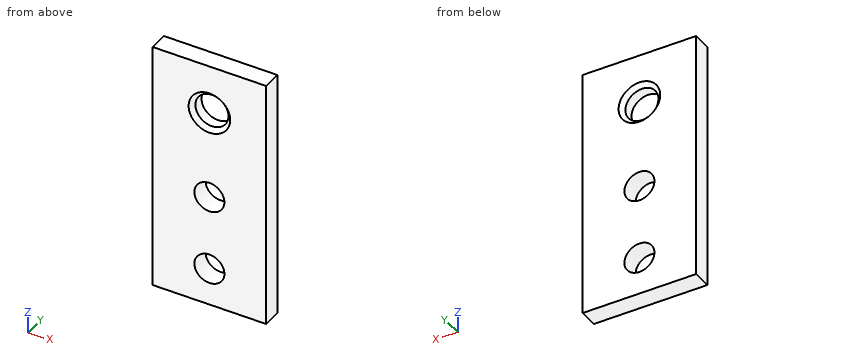
```python
from build123d import *

# Parameters (mm, degrees)
SKETCH1_W                   = 38.1
SKETCH1_H                   = 6.35
EXTRUDE1_DEPTH              = 84.455
F_3_8_CLEARANCE_HOLE1_D     = 10.0838
F_3_8_CLEARANCE_HOLE1_DEPTH = 16.002
F_3_8_CLEARANCE_HOLE1_TIP   = 3.029479155


with BuildPart() as part:
    # Sketch1 → Extrude1 (new body)
    with BuildSketch(Plane.XY):
        Rectangle(SKETCH1_W, SKETCH1_H)
    extrude(amount=EXTRUDE1_DEPTH)

    # 3/8 Clearance Hole1
    with Locations(Plane(origin=(0, 3.175, 12.7), x_dir=(0, 0, 1), z_dir=(0, 1, 0))):
        with Locations((0, 0), (25.4, 0)):
            Hole(F_3_8_CLEARANCE_HOLE1_D / 2, depth=F_3_8_CLEARANCE_HOLE1_DEPTH)
            with Locations((0, 0, -(F_3_8_CLEARANCE_HOLE1_DEPTH + F_3_8_CLEARANCE_HOLE1_TIP / 2))):  # 118° drill point
                Cone(0, F_3_8_CLEARANCE_HOLE1_D / 2, F_3_8_CLEARANCE_HOLE1_TIP, mode=Mode.SUBTRACT)

    # Sketch4 → 7/16 (0.4375) Diameter Hole2 (revolve, cut)
    with BuildSketch(Plane(origin=(0, 3.175, 67.945), x_dir=(0, 0, 1), z_dir=(1, 0, 0))):
        Polygon((0, 0), (0, 6.35), (6.985, 6.35), (5.55625, 4.92125), (5.55625, 1.42875), (6.985, 0), align=None)
    revolve(axis=Axis((0, 9.525, 67.945), (0, -1, 0)), mode=Mode.SUBTRACT)


solid = part.part
```
The listing builds one solid part. Answer for the finished solid, in the listing's coordinates (mm). Give positions to 0.01 mm unless a question says otherwise; leave off trailing zeros. Loops run counter-clockwise (first coordinate to the right, second up) from the corner with the lowest first, then second, coordinate; pieces in that order, holes last. Notation, with made-up numbers: (84.25, -18.5) - (114.25, -18.5) arc R14 ccw to (114.25, 8.5) - close; hole circle Ø5 at (8, -2.75). An arc over 180 degrees is marked (long way). Answer as CSV lines item,"result". Start each with the question number.
Item 1: A cutting plane is placed at B-B on z = 38.1. Determine the outline of the cut face in (x, y) (3 decimals), then the cut area to 3 significant figures.
Item 2: A cutting plane is placed at C-C on y = -0.25. Count the separate pieces of the cut face and the enclosed holes in it, then the cut area to 3 significant figures.
Item 3: A cutting plane is placed at A-A on x = 0. Determine the outline of the cut face in (y, z) (3 decimals).
Item 4: This flat-tipped pin is pushed along its axis until it touches: pin 1 (6 mm diameter, centred on x = 0, z = 38.1, fed in from -Y). Where does it stop, or does it pass through?
Item 5: Find the intervals of material crossed by line 1 (X direction, y = 1.5, z = 12.7); line 2 (X direction, y = 1.75, z = 72), in increasing order. Write a range as from..to.
Found:
1,outline,"(-19.05, -3.175) - (-5.042, -3.175) - (-5.042, 3.175) - (-19.05, 3.175) - close; (5.042, -3.175) - (19.05, -3.175) - (19.05, 3.175) - (5.042, 3.175) - close"
1,area,"178 mm^2"
2,separate pieces,"1"
2,enclosed holes,"3"
2,area,"2,960 mm^2"
3,outline,"(-3.175, 0) - (3.175, 0) - (3.175, 7.658) - (-3.175, 7.658) - close; (-3.175, 17.742) - (3.175, 17.742) - (3.175, 33.058) - (-3.175, 33.058) - close; (-3.175, 43.142) - (3.175, 43.142) - (3.175, 60.96) - (1.746, 62.389) - (-1.746, 62.389) - (-3.175, 60.96) - close; (-3.175, 74.93) - (-1.746, 73.501) - (1.746, 73.501) - (3.175, 74.93) - (3.175, 84.455) - (-3.175, 84.455) - close"
4,pin 1,"passes through"
5,line 1,"x = -19.05..-5.04, 5.04..19.05"
5,line 2,"x = -19.05..-3.8, 3.8..19.05"
